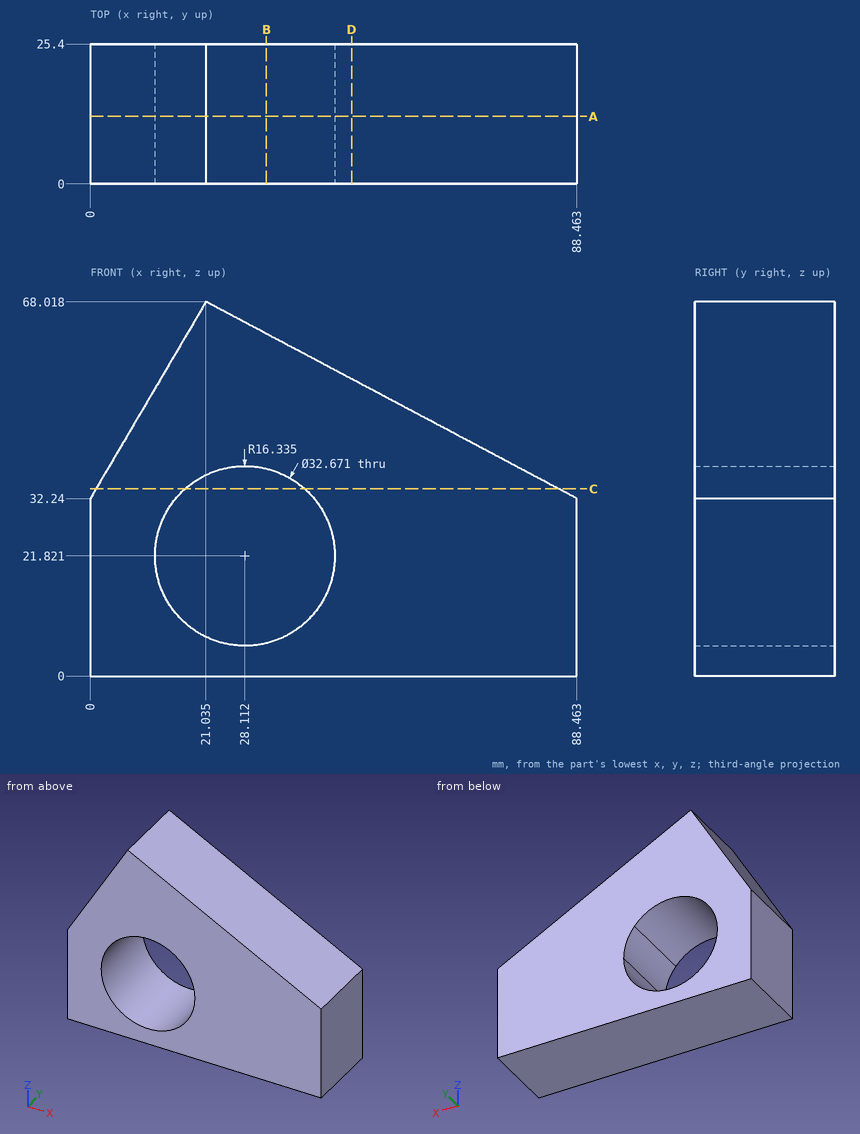
Check sheet for the drawn part. Datum: minimum x, y, z corner. Units: mm. Give positions to 0.01 mm unless a question says otherwise; leave off trailing zeros. Order: outer loops, then holes, each group sorted by start corner. A loop starts at its lowest first (then second) coordinate and runs counter-clockwise, first axis right, second up. Notation, with made-up numbers: (6.5, -2) - (43.5, -2) arc R22 ccw to (43.5, 25) - close; hole circle Ø10 at (-8, 9.25). An arc over 180 degrees is marked (long way). Answer in a Markdown table with one row per item. Add a question column.
Q1. Material ranges on probe 1 along Z at (x, y) = (22, 20.5) (1 decimal); probe 2 along X at (y, z) = (15, 28) (1 decimal); probe 3 along Z at (x, y) = (40, 18.25) (1 decimal), recorded low to high. Write a range as from..to.
Q2. Gauge pin test, flat ends, axial feed: pin 1 (4 mm diameter, centred on x = 47.5, y = 6, fed in from +Z); pin 2 (8 mm diameter, centred on y = 16, z = 49.5, fed in from +X) (1 decimal); pin 3 (1.5 mm diameter, centred on x = 50, y = 7.5, fed in from +Z). Record the tip position at first contact, or that the pin passes through.
Q3. Cross-section at C-C, the plane z = 34. Enter the section's corners in (x, y) (1 decimal).
Q4. Cross-section at A-A, the plane y = 12.25. Enter the section's corners in (x, z) (1 decimal), then the cut area to 3 significant figures.
Q5. Cross-section at D-D, the plane x = 47.5. Enter the section's corners in (y, z) (1 decimal).
Q6. Cross-section at B-B, the plane x = 32. Enter the section's corners in (y, z) (1 decimal).
Check values:
| question | item | result |
|---|---|---|
| 1 | probe 1 | z = 0..6.7, 37..67.5 |
| 1 | probe 2 | x = 0..13, 43.2..88.5 |
| 1 | probe 3 | z = 0..10.6, 33..58 |
| 2 | pin 1 | stops at z = 55.04 |
| 2 | pin 2 | stops at x = 63.5 |
| 2 | pin 3 | stops at z = 53.05 |
| 3 | outline | (1, 0) - (17.2, 0) - (17.2, 25.4) - (1, 25.4) - close; (39, 0) - (85.1, 0) - (85.1, 25.4) - (39, 25.4) - close |
| 4 | outline | (0, 0) - (88.5, 0) - (88.5, 32.2) - (21, 68) - (0, 32.2) - close; hole circle Ø32.7 at (28.1, 21.8) |
| 4 | area | 3,600 mm^2 |
| 5 | outline | (0, 0) - (25.4, 0) - (25.4, 54) - (0, 54) - close |
| 6 | outline | (0, 0) - (25.4, 0) - (25.4, 6) - (0, 6) - close; (0, 37.7) - (25.4, 37.7) - (25.4, 62.2) - (0, 62.2) - close |
